Can you work these out from the model? Positions are in its coordinate system, mm. Face numbers are marked on the shaded views. A direction names the side the tool comes from. Give positions to 0.01 mm unless a question says otherwise; leave off trailing zeros. Write each loop counter-clockwise with the first axis right and the second up, starting at its lowest first coordinate (ties: lowest second). Pieces come first, ordered by that corner, then holes. Notation, with made-up numbers: (-5, 1) -> (39, 1) arc R8 ccw to (39, 15) -> close; hole circle Ø5 at (54, 48). An arc over 180 degrees is marked (long way). Answer as CSV lines item,"result". Start each with the question number.
1. I'm going to push flat-ended pins straight in: P1, Ø6, axis at x = -35.5, z = -4.5, coming from the +Y side; P2, Ø1.5, axis at x = 19, y = -16.5, coming from the +Z side. Where does each tip first touch, or does it pass through?
2. If we mould it in two halves opening along X, with no side actions, what happens to the marked faces 1, 2 and 3? For each: pulls with the +X half, pulls with the -X half, needs draft (parallel to the pull), parting line crosses it, or undercut.
3. If we section it at B-B on z = -5: Write out the boundary of the cut face in (x, y), plus the area to 3 significant figures.
4. I need wall thicknesses on line 1 (X direction, y = -5.75, z = 24); line 2 (X direction, y = -25.5, z = -3); line 3 (X direction, y = -6.75, z = 22). Which ranges of each line are inside material? Lowest first, please. Write a range as [from, to].
5. If we section it at A-A on x = -28: Write out the boundary of the cut face in (y, z).
6. On a 3-axis mill with a long thin cutter (end or side, diameter ignored), from which of +Z, -Z, +X, -X, +Y, -Y can I reach the whole of each face in a straight line? I mean the marked faces 4 and 5. Say none if no direction works.
7. If we section it at D-D on z = 13.5: Write out the boundary of the cut face in (x, y), plus the area to 3 significant figures.
8. If we section it at C-C on y = -15: Write out the boundary of the cut face in (x, z), plus the area to 3 significant figures.
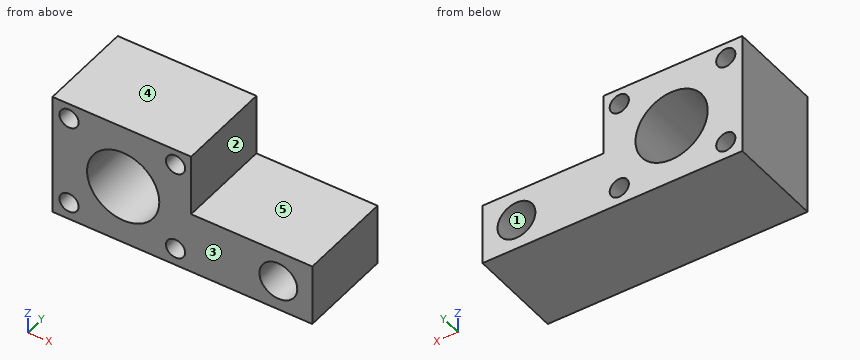
```python
from build123d import *

# Parameters (mm, degrees)
F0_R     = 3
F0_R_2   = 11.309241
F0_R_3   = 5.923824
F1_DEPTH = 30


with BuildPart() as f1:
    # F0 (on Front) → F1 (new body)
    with BuildSketch(Plane.XZ):
        Polygon((-8.18941, 29.022118), (-51.57891, 29.022118), (-51.57891, -9.482474), (-8.18941, -9.482474), (29.740484, -9.482474), (29.740484, 9.769822), (-8.18941, 9.769822), align=None)
        with Locations((-46.406654, -4.022868)):
            Circle(F0_R, mode=Mode.SUBTRACT)
        with Locations((-13.074319, -4.022868)):
            Circle(F0_R, mode=Mode.SUBTRACT)
        with Locations((-29.453138, 9.195126)):
            Circle(F0_R_2, mode=Mode.SUBTRACT)
        with Locations((19.108622, 0)):
            Circle(F0_R_3, mode=Mode.SUBTRACT)
        with Locations((-46.406654, 24.137207)):
            Circle(F0_R, mode=Mode.SUBTRACT)
        with Locations((-13.074319, 24.137207)):
            Circle(F0_R, mode=Mode.SUBTRACT)
    extrude(amount=F1_DEPTH)


solid = f1.part
```
Computed values:
1,P1,"stops at y = 0"
1,P2,"stops at z = 9.77"
2,face 1,"undercut"
2,face 2,"pulls with the +X half"
2,face 3,"needs draft"
3,outline,"(-51.58, -30) -> (-49.24, -30) -> (-49.24, 0) -> (-51.58, 0) -> close; (-43.57, -30) -> (-15.91, -30) -> (-15.91, 0) -> (-43.57, 0) -> close; (-10.24, -30) -> (15.93, -30) -> (15.93, 0) -> (-10.24, 0) -> close; (22.29, -30) -> (29.74, -30) -> (29.74, 0) -> (22.29, 0) -> close"
3,area,"1,910 mm2"
4,line 1,"x = [-51.58, -49.4], [-43.41, -16.07], [-10.08, -8.19]"
4,line 2,"x = [-51.58, -49.23], [-43.59, -15.89], [-10.25, 14], [24.22, 29.74]"
4,line 3,"x = [-51.58, -48.51], [-44.3, -15.18], [-10.97, -8.19]"
5,outline,"(-30, -9.48) -> (0, -9.48) -> (0, -2.02) -> (-30, -2.02) -> close; (-30, 20.41) -> (0, 20.41) -> (0, 29.02) -> (-30, 29.02) -> close"
6,face 4,"+Z, +X, -X, +Y, -Y"
6,face 5,"+Z, +X, +Y, -Y"
7,outline,"(-51.58, -30) -> (-39.91, -30) -> (-39.91, 0) -> (-51.58, 0) -> close; (-19, -30) -> (-8.19, -30) -> (-8.19, 0) -> (-19, 0) -> close"
7,area,"674 mm2"
8,outline,"(-51.58, -9.48) -> (29.74, -9.48) -> (29.74, 9.77) -> (-8.19, 9.77) -> (-8.19, 29.02) -> (-51.58, 29.02) -> close; hole circle Ø6 at (-46.41, -4.02); hole circle Ø6 at (-46.41, 24.14); hole circle Ø22.62 at (-29.45, 9.2); hole circle Ø6 at (-13.07, -4.02); hole circle Ø6 at (-13.07, 24.14); hole circle Ø11.85 at (19.11, 0)"
8,area,"1,780 mm2"
